Design review of the part built by this model. Coordinates are the model's own, in mm. A direction names the side the tool comes from. Round coordinates to 2 decimals unless told otherwise and drop trailing zeros. Write each loop counter-clockwise with the first axis right and the second up, starting at its lowest first coordinate (ties: lowest second). Pieces come first, ordered by that corner, then holes. Notation, with made-up numbers: M 47.25,79.5 L 84.25,79.5 A16 cw 84.25,88.5 Z; hole C -11,31.25 d8. An arc over 180 degrees is marked long. Use CSV: the item, a comma, the result in double quotes.
Autodesk Inventor part; units mm, degrees
ref_plane "YZ Plane" through (0, 0, 0) normal (1, 0, 0) x (0, 1, 0)
ref_plane "XZ Plane" through (0, 0, 0) normal (0, 1, 0) x (-1, 0, 0)
ref_plane "XY Plane" through (0, 0, 0) normal (0, 0, 1) x (1, 0, 0)
sketch "Sketch1" plane through (0, 0, 0) normal (0, 0, 1) x (1, 0, 0)
  line L0 (0, 0) -> (0, 25.4)
  line L1 (0, 0) -> (5.969, 0)
  line L2 (5.969, 0) -> (5.969, 25.4)
  arc A0 (0, 25.4) -> (5.969, 25.4) centre (2.9845, 27.0884) ccw
  dimension "d0" = 3.429
  dimension "d1" = 25.4
  dimension "d2" = 5.969
revolve "Revolution1" add sketch "Sketch1" angle 360 about axis through (0, 0, 0) along (1, 0, 0)
sketch "Sketch2" plane through (5.969, 0, 0) normal (1, 0, 0) x (0, 0, -1)
  circle A0 centre (0, 0) radius 26.9875
  dimension "d4" = 53.975
extrude "Extrusion1" add sketch "Sketch2" along normal blind 3.175
sketch "Sketch3" plane through (0, 0, 0) normal (-1, 0, 0) x (0, 0, 1)
  circle A0 centre (0, 0) radius 26.9875
  dimension "d7" = 53.975
extrude "Extrusion2" add sketch "Sketch3" along normal blind 3.175
sketch "Sketch4" plane through (-3.175, 0, 0) normal (-1, 0, 0) x (0, 0, 1)
  circle A0 centre (0, 0) radius 14.2875
  dimension "d10" = 28.575
extrude "Extrusion3" cut sketch "Sketch4" against normal through all
fillet "Fillet1" radius 0.9525 2 edges at (-3.175, 0, -26.9875) (9.144, 0, 26.9875)
properties part number "1 1_8 Bore Pollycord Pully" material "ABS Plastic"
1) Add section D-D on x = 2.75. Write out the cut boundary in (y, z) (1 decimal).
Answers:
outline,"C 0,0 d47.3; hole C 0,0 d28.6"
2) The part is to be moulded in two halves that separate along Y. For faces 3 (the face through (5.969, -16, -20)), 4 (the face through (2.898, 0.628, -14.274)), 5 (the face through (-1.1, -18.24, -19.89)), say which applies: released by +Y, released by -Y, zero draft, split by the parting line, or undercut.
Answers:
face 3,"zero draft"
face 4,"undercut"
face 5,"split by the parting line"
3) For pin 1 Ø2 at (x, z) = (8, 6) entering from +Y; pin 2 Ø5 at (x, y) = (5.5, -17) entering from -Z; pin 3 Ø3 at (x, z) = (7, 14) entering from -Y, all flat-tipped, find the tip position at first contact; note any pin that passes through.
Answers:
pin 1,"y = 26.52"
pin 2,"z = -22.73"
pin 3,"y = -23.92"
4) Add section C-C on x = 6.75. Write out the cut boundary in (y, z) (1 decimal).
Answers:
outline,"C 0,0 d54; hole C 0,0 d28.6"
5) Wall thickness on line 1 along X through (y, z) = (19.5, 17) (3 decimals); line 2 along Y through (x, z) = (4.75, -3); line 3 along Y through (x, z) = (0.5, -4): over which ranges is each line inside the solid? List them lowest first. Write a range as [from, to].
Answers:
line 1,"[-3.175, 0], [5.969, 9.144]"
line 2,"[-23.96, -13.97], [13.97, 23.96]"
line 3,"[-24.4, -13.72], [13.72, 24.4]"
6) Machinability: for faces 1 (the face through (-3.175, -11, 11)), 2 (the face through (0, -16, 20)), which of the approach directions +Z, -Z, +X, -X, +Y, -Y give a long, thin tool a straight path to every point of the face, cutting with its end or side? Answer none if there is none.
Answers:
face 1,"+Z, -Z, -X, +Y, -Y"
face 2,"none"
7) Add section A-A on y = 0. Write out the cut boundary in (x, z) (1 decimal).
Answers:
outline,"M -3.2,-26 A1 ccw -2.2,-27 L 0,-27 L 0,-25.4 A3.4 cw 6,-25.4 L 6,-27 L 8.2,-27 A1 ccw 9.1,-26 L 9.1,-14.3 L -3.2,-14.3 Z; M -3.2,14.3 L 9.1,14.3 L 9.1,26 A1 ccw 8.2,27 L 6,27 L 6,25.4 A3.4 cw 0,25.4 L 0,27 L -2.2,27 A1 ccw -3.2,26 Z"
